from build123d import *

# Parameters (mm, degrees)
BOSS_EXTRUDE1_DEPTH = 2.4


with BuildPart() as part:
    # Sketch1 → Boss-Extrude1 (new body)
    with BuildSketch(Plane.XY):
        with BuildLine():
            Line((-76.2, -12.7), (-76.2, -2.4))
            Line((-76.2, -2.4), (-73.8, -2.4))
            Line((-73.8, -2.4), (-73.8, 10.3))
            Line((-73.8, 10.3), (-76.2, 10.3))
            Line((-76.2, 10.3), (-76.2, 23))
            Line((-76.2, 23), (-73.8, 23))
            Line((-73.8, 23), (-73.8, 35.7))
            Line((-73.8, 35.7), (-76.2, 35.7))
            Line((-76.2, 35.7), (-76.2, 48.4))
            Line((-76.2, 48.4), (-73.8, 48.4))
            Line((-73.8, 48.4), (-73.8, 61.1))
            Line((-73.8, 61.1), (-76.2, 61.1))
            Line((-76.2, 61.1), (-76.2, 63.5))
            Line((-76.2, 63.5), (-63.5, 63.5))
            Line((-63.5, 63.5), (-63.5, 61.1))
            Line((-63.5, 61.1), (-50.8, 61.1))
            Line((-50.8, 61.1), (-50.8, 63.5))
            Line((-50.8, 63.5), (-38.1, 63.5))
            Line((-38.1, 63.5), (-38.1, 61.1))
            Line((-38.1, 61.1), (-25.4, 61.1))
            Line((-25.4, 61.1), (-25.4, 63.5))
            Line((-25.4, 63.5), (-12.7, 63.5))
            Line((-12.7, 63.5), (-12.7, 61.1))
            Line((-12.7, 61.1), (-0.428418776, 61.1))
            Line((-0.428418776, 61.1), (3.875889615, 59.512715672))
            Line((3.875889615, 59.512715672), (4.706267152, 61.764486785))
            Line((4.706267152, 61.764486785), (16.621889293, 57.370405654))
            Line((16.621889293, 57.370405654), (15.791511757, 55.118634541))
            Line((15.791511757, 55.118634541), (27.707133898, 50.72455341))
            Line((27.707133898, 50.72455341), (28.537511435, 52.976324523))
            Line((28.537511435, 52.976324523), (40.453133576, 48.582243393))
            Line((40.453133576, 48.582243393), (39.622756039, 46.330472279))
            Line((39.622756039, 46.330472279), (51.538378181, 41.936391148))
            Line((51.538378181, 41.936391148), (52.368755717, 44.188162262))
            Line((52.368755717, 44.188162262), (64.284377859, 39.794081131))
            Line((64.284377859, 39.794081131), (63.454000322, 37.542310018))
            Line((63.454000322, 37.542310018), (75.369622463, 33.148228887))
            Line((75.369622463, 33.148228887), (76.2, 35.4))
            Line((76.2, 35.4), (76.2, 10))
            Line((76.2, 10), (63.5, 10))
            Line((63.5, 10), (63.5, 12.4))
            Line((63.5, 12.4), (50.8, 12.4))
            Line((50.8, 12.4), (50.8, 10))
            Line((50.8, 10), (38.1, 10))
            Line((38.1, 10), (38.1, 12.4))
            Line((38.1, 12.4), (25.4, 12.4))
            Line((25.4, 12.4), (25.4, 10))
            Line((25.4, 10), (12.7, 10))
            Line((12.7, 10), (12.7, 12.4))
            Line((12.7, 12.4), (0, 12.4))
            Line((0, 12.4), (0, 10))
            Line((0, 10), (0, 9.525))
            ThreePointArc((0, 9.525), (-9.525, 0), (0, -9.525))
            Line((0, -9.525), (0, -12.7))
            Line((0, -12.7), (-76.2, -12.7))
        make_face()
    extrude(amount=BOSS_EXTRUDE1_DEPTH)


solid = part.part
The listing builds one solid part. Answer for the finished solid, in the listing's coordinates (mm). Round coordinates to 2 decimals unless told otherwise and drop trailing zeros. Order: outer loops, then holes, each group sorted by start corner. A loop starts at its lowest first (then second) coordinate and runs counter-clockwise, first axis right, second up. Notation, with made-up numbers: (83.25, 16.5) -> (111.25, 16.5) arc R38 cw to (111.25, 55.5) -> close; hole circle Ø2 at (-39.5, 19). An arc over 180 degrees is marked (long way). Put each result on its own line as item: value.
Q1. Determine the mould class of faces 1 (the flat face through (34.41, 50.81, 1.18)), 2 (the flat face through (45.497, 44.164, 1.183)), 3 (the flat face through (-16, 26, 0)) for opening direction X: pulls with the +X half, pulls with the -X half, needs draft (parallel to the pull), parting line crosses it, or undercut.
Results list:
face 1: pulls with the +X half
face 2: undercut
face 3: needs draft
Q2. Consider line 1 along X through (y, z) = (10.5, 1.9); line 2 along X through (y, z) = (29.5, 2.25); line 3 along Y through (x, z) = (-56, 1.3). Determine where each line is inside the solid, lowest interval first.
Results list:
line 1: -76.2 to 0, 12.7 to 25.4, 38.1 to 50.8, 63.5 to 76.2
line 2: -73.8 to 76.2
line 3: -12.7 to 61.1
Q3. Each of these flat-tipped pins is pushed along its axis until it touches: P1, Ø0.7, axis at y = 4.5, z = 1, coming from the -X side; P2, Ø0.7, axis at x = -54, z = 0.5, coming from the +Y side; P3, Ø4, axis at x = -39, y = 21.5, coming from the -Z side; P4, Ø1.2, axis at x = 34, z = 1, coming from the -Y side. Where does it stop, or does it pass through?
Results list:
P1: x = -73.8
P2: y = 61.1
P3: z = 0
P4: y = 12.4
Q4. Section B-B, the plane y = 0 is taken. Write down the section's boundary in (x, z) (3 decimals), and give its area (3 significant figures).
Results list:
outline: (-73.8, 0) -> (-9.525, 0) -> (-9.525, 2.4) -> (-73.8, 2.4) -> close
area: 154 mm^2
Q5. Section A-A, the plane x = -6 is taken. Write down the section's boundary in (y, z).
Results list:
outline: (-12.7, 0) -> (-7.4, 0) -> (-7.4, 2.4) -> (-12.7, 2.4) -> close; (7.4, 0) -> (61.1, 0) -> (61.1, 2.4) -> (7.4, 2.4) -> close
Q6. Section C-C, the plane x = 44 is taken. Write down the section's boundary in (y, z), and give its area (3 significant figures).
Results list:
outline: (10, 0) -> (44.72, 0) -> (44.72, 2.4) -> (10, 2.4) -> close
area: 83.3 mm^2
